from build123d import *

# Parameters (mm, degrees)
SKETCH_1_R               = 6
EXTRUDE_1_DEPTH          = 43
SKETCH_2_OUTSIDE_W       = 23.246
SKETCH_2_OUTSIDE_H       = 23.246
SKETCH_2_OUTSIDE_R       = 5.5
CUT_EXTRUDE_1_DEPTH      = 6
CUT_EXTRUDE_2_DEPTH      = 44.829214002
CUT_EXTRUDE_2_DEPTH_BACK = 44.829214002
CUT_EXTRUDE_START        = -3.5
CUT_EXTRUDE_3_DEPTH      = 41.329214002


# Read off the part's stored shape, not the designer's step: 替换面1
with BuildPart() as part:
    # 草图1 → 凸台-拉伸1 (new body)
    with BuildSketch(Plane.XY):
        Circle(SKETCH_1_R)
    extrude(amount=EXTRUDE_1_DEPTH)

    # 草图2 outside → 切除-拉伸1 (cut)
    with BuildSketch(Plane.XY.offset(43)):
        Rectangle(SKETCH_2_OUTSIDE_W, SKETCH_2_OUTSIDE_H)
        Circle(SKETCH_2_OUTSIDE_R, mode=Mode.SUBTRACT)
    extrude(amount=-CUT_EXTRUDE_1_DEPTH, mode=Mode.SUBTRACT)

    # 替换面1 outline → 替换面1 (revolve, cut)
    with BuildSketch(Plane.XZ):
        with BuildLine():
            ThreePointArc((0, 43), (2.870847837, 42.579051764), (5.500000008, 41.351646539))
            Line((5.500000008, 41.351646539), (5.500000008, 43))
            Line((5.500000008, 43), (0, 43))
        make_face()
    revolve(axis=Axis((0, 0, 0), (0, 0, 1)), mode=Mode.SUBTRACT)

    # 草图5 → 切除-拉伸2 (cut, two sides: drawn at the far end of the back side and taken through both)
    with BuildSketch(Plane(origin=(0, 0, 0), x_dir=(0, 0, -1), z_dir=(1, 0, 0)).offset(-CUT_EXTRUDE_2_DEPTH_BACK)):
        Polygon((20.642732015, -103.11641858), (0, -6), (-2.55067874, 6), (-23.193410755, 103.11641858), (171.039426405, 144.40188261), (214.875569175, -61.83095455), align=None)
    extrude(amount=CUT_EXTRUDE_2_DEPTH + CUT_EXTRUDE_2_DEPTH_BACK, mode=Mode.SUBTRACT)

    # 草图6 → 切除-拉伸3 (cut, through all)
    with BuildSketch(Plane(origin=(0, 0, 0), x_dir=(0, 0, -1), z_dir=(1, 0, 0)).offset(CUT_EXTRUDE_START)):
        with BuildLine():
            Line((-15, -2.5), (-23, -2.5))
            ThreePointArc((-23, -2.5), (-25.5, 0), (-23, 2.5))
            Line((-23, 2.5), (-15, 2.5))
            ThreePointArc((-15, 2.5), (-12.5, 0), (-15, -2.5))
        make_face()
    extrude(amount=-CUT_EXTRUDE_3_DEPTH, mode=Mode.SUBTRACT)


solid = part.part
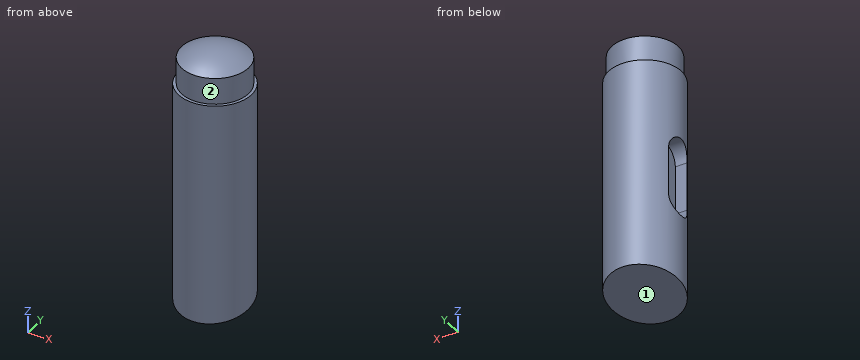
For this review, take the finished solid that the model builds, in its own axes (mm). Face numbers are marked on the shaded views. A direction names the side the tool comes from. Round coordinates to 2 decimals unless told otherwise and drop trailing zeros. Loops run counter-clockwise (first coordinate to the right, second up) from the corner with the lowest first, then second, coordinate; pieces in that order, holes last. Notation, with made-up numbers: (46.25, 73.5) - (94.25, 73.5) arc R32 cw to (94.25, 109.5) - close; hole circle Ø3 at (-38.75, 86). An arc over 180 degrees is marked (long way). One line per item, written item: value. Start each with the question number.
Item 1: For the marked faces 1 and 2, list the 3-axis set-ups (+Z, -Z, +X, -X, +Y, -Y) from which the entire face can be reached by the end or side of a thin tool; tool diameter is ignored.
Item 2: Take a section at B-B (y = 0.5). Give the boundary of the cut face in (x, z).
Item 3: For L1, parallel to Z at x = -2.5, y = 2.5; L2, parallel to Y at x = -1, z = 27.5; L3, parallel to Y at x = 4, z = 23.5, list the stretches that pass through material, from the lowest coordinate up.
Item 4: Take a section at C-C (x = -1.5). Give the boundary of the cut face in (y, z), plus the area to 3 significant figures.
Item 5: Clearance check with flat-ended pins moving along their axes: pin 1 Ø1 at (x, z) = (1, 24) entering from -Y; pin 2 Ø6 at (y, z) = (4, 22) entering from +X; pin 3 Ø6 at (y, z) = (-4.5, 19.5) entering from +X; pin 4 Ø6 at (x, z) = (-1.5, 6.5) entering from +Y. State where each tip first meets the part, or that it passes through.
Item 6: Take a section at A-A (z = 31). Give the boundary of the cut face in (x, y).
Item 7: Take a section at D-D (z = 22). Give the boundary of the cut face in (x, y), plus the area to 3 significant figures.
Answer below:
1. face 1: -Z, +X, -X, +Y
1. face 2: +Z
2. outline: (-5.98, 1.38) - (5.98, 1.38) - (5.98, 37) - (5.48, 37) - (5.48, 41.35) arc R9.99 ccw to (-5.48, 41.35) - (-5.48, 37) - (-5.98, 37) - (-5.98, 25.45) - (-3.5, 25.45) - (-3.5, 12.55) - (-5.98, 12.55) - close
3. L1: z = 1.81 to 42.35
3. L2: y = -5.92 to 5.92
3. L3: y = -4.47 to 4.47
4. outline: (-5.81, 0.04) - (5.81, 2.51) - (5.81, 37) - (5.29, 37) - (5.29, 41.35) arc R9.89 ccw to (-5.29, 41.35) - (-5.29, 37) - (-5.81, 37) - close
4. area: 472 mm2
5. pin 1: stops at y = -5.98
5. pin 2: stops at x = 5.92
5. pin 3: stops at x = 5.81
5. pin 4: stops at y = 6
6. outline: circle Ø12 at (0, 0)
7. outline: (-5.45, -2.5) arc R6 ccw (long way) to (-5.45, 2.5) - (-3.5, 2.5) - (-3.5, -2.5) - close
7. area: 101 mm2
